Input: part model. Units: mm. Frame: model coordinates. A direction names the side the tool comes from. Give positions to 0.01 mm unless a question says otherwise; leave off trailing zeros. Order: outer loops, then holes, each group sorted by start corner. A loop starts at its lowest first (then second) coordinate and runs counter-clockwise, first axis right, second up. Notation, with made-up numbers: (20.25, 9) - (48.25, 9) arc R18 cw to (48.25, 20) - close; hole circle Ø5 at (29.25, 76). An arc over 180 degrees is marked (long way). Use a Markdown table: item, result.
from build123d import *

# Parameters (mm, degrees)
F0_R          = 46.05
F1_DEPTH      = 15.24
F2_R          = 45.75
F3_DEPTH      = 12.7
F4_R          = 4.1
F5_DEPTH      = 3.53
F5_DEPTH_BACK = 1
F7_DEPTH      = 15.241
F8_R          = 3.1
F9_DEPTH      = 18.771


# Not quite as in the source:
# - after a boolean that leaves OpenCascade's solid faulty, fix() repairs it


with BuildPart() as f1:
    # F0 (on Top) → F1 (new body)
    with BuildSketch(Plane.XY):
        Circle(F0_R)
    extrude(amount=F1_DEPTH)

    # F2 (on Top) → F3 (cut)
    with BuildSketch(Plane.XY):
        Circle(F2_R)
    extrude(amount=F3_DEPTH, mode=Mode.SUBTRACT)

    # F4 (on face) → F5 (join, two sides)
    with BuildSketch(Plane.XY.offset(15.24)) as f5_sk:
        Circle(F4_R)
    extrude(amount=F5_DEPTH)
    extrude(f5_sk.sketch, amount=-F5_DEPTH_BACK)

    # F6 (on face) → F7 (cut, through all)
    with BuildSketch(Plane.XY.offset(15.24)):
        with BuildLine():
            Line((0, 4.1), (0, 46.03))
            ThreePointArc((0, 46.03), (-46.03, 0), (0, -46.03))
            Line((0, -46.03), (0, -4.1))
            ThreePointArc((0, -4.1), (-4.1, 0), (0, 4.1))
        make_face()
    extrude(amount=-F7_DEPTH, mode=Mode.SUBTRACT)

    add(f1.part.fix(), mode=Mode.REPLACE)

    # F8 (on face) → F9 (cut, through all)
    with BuildSketch(Plane.XY.offset(18.77)):
        Circle(F8_R)
    extrude(amount=-F9_DEPTH, mode=Mode.SUBTRACT)


solid = f1.part
1. Pin query (flat end, axial travel): pin 1 (7.5 mm diameter, centred on y = -19.5, z = 6.5, fed in from -X); pin 2 (6 mm diameter, centred on x = -11, z = 15.5, fed in from +Y); pin 3 (3 mm diameter, centred on x = -15.5, z = 7.5, fed in from -Y). Return the tip coordinate at first contact, or that it passes through.
Response:
| item | result |
|---|---|
| pin 1 | stops at x = -43.27 |
| pin 2 | stops at y = 45.35 |
| pin 3 | stops at y = -43.87 |
2. Set-up query: faces 1 (the face through (45.74, -1.01, 6.26)), 2 (the face through (0, 25, 14)). Return all of +Z, -Z, +X, -X, +Y, -Y with unobstructed straight access to the full face (end or side cutting, diameter ignored); none if empty.
Response:
| item | result |
|---|---|
| face 1 | -Z |
| face 2 | +Z, -Z |
3. Mould query, pull axis X, two halves, no side actions, for faces 3 (the face through (21.249, -40.854, 7.513)), 4 (the face through (20, 1, 12.7)), 5 (the face through (-2, 3, 18.77)). Classes: pulls with the +X half, pulls with the -X half, needs draft (parallel to the pull), parting line crosses it, or undercut.
Response:
| item | result |
|---|---|
| face 3 | parting line crosses it |
| face 4 | undercut |
| face 5 | needs draft |
4. Section query A-A (y = 0). State how many separate pieces and enclosed holes the cut face has, then the cut area to 3 significant figures.
Response:
| item | result |
|---|---|
| separate pieces | 3 |
| enclosed holes | 0 |
| area | 123 mm^2 |
5. Section query C-C (z = 10). Return loops of the section in (x, y), then the cut area to 3 significant figures.
Response:
| item | result |
|---|---|
| outline | circle Ø92.1 at (0, 0); hole (0, -46.03) - (0, -45.75) arc R45.75 ccw to (0, 45.75) - (0, 46.03) arc R46.03 ccw to start |
| area | 46.2 mm^2 |
6. Material intervals for line 1 along Y through (x, z) = (0, 16.5); line 2 along Y through (x, z) = (14, 3.5); line 3 along Z through (x, y) = (10.5, -7.5), sorted ascending.
Response:
| item | result |
|---|---|
| line 1 | y = -4.1 to -3.1, 3.1 to 4.1 |
| line 2 | y = -43.87 to -43.56, 43.56 to 43.87 |
| line 3 | z = 12.7 to 15.24 |
